Autodesk Inventor part; units mm, degrees
ref_plane "YZ Plane" through (0, 0, 0) normal (1, 0, 0) x (0, 1, 0)
ref_plane "XZ Plane" through (0, 0, 0) normal (0, 1, 0) x (-1, 0, 0)
ref_plane "XY Plane" through (0, 0, 0) normal (0, 0, 1) x (1, 0, 0)
sketch "Sketch1" plane through (0, 0, 0) normal (0, 1, 0) x (-1, 0, 0)
  line L0 (16.2, 12.4) -> (-16.2, 12.4)
  line L1 (-16.2, 12.4) -> (-16.2, -12.4)
  line L2 (-16.2, -12.4) -> (16.2, -12.4)
  line L3 (16.2, -12.4) -> (16.2, 12.4)
  line L4 (16.2, 12.4) -> (-16.2, -12.4) construction
  line L5 (-16.2, 12.4) -> (16.2, -12.4) construction
  point P0 (0, 0)
  dimension "d0" = 32.4
  dimension "d1" = 24.8
extrude "Extrusion1" add sketch "Sketch1" against normal blind 1.4
sketch "Sketch2" plane through (0, 0, 0) normal (0, 1, 0) x (1, 0, 0)
  line L0 (-18, -14) -> (18, -14)
  line L1 (18, -14) -> (18, 14)
  line L2 (18, 14) -> (-18, 14)
  line L3 (-18, 14) -> (-18, -14)
  line L4 (-18, -14) -> (18, 14) construction
  line L5 (18, -14) -> (-18, 14) construction
  point P0 (0, 0)
  dimension "d4" = 36
  dimension "d5" = 28
extrude "Extrusion2" add sketch "Sketch2" along normal blind 2
sketch "Sketch3" plane through (0, 2, 0) normal (0, 1, 0) x (1, 0, 0)
  line L0 (-8.5, -9) -> (8.5, -9)
  line L1 (8.5, -9) -> (8.5, 9)
  line L2 (8.5, 9) -> (-8.5, 9)
  line L3 (-8.5, 9) -> (-8.5, -9)
  line L4 (-8.5, -9) -> (8.5, 9) construction
  line L5 (8.5, -9) -> (-8.5, 9) construction
  circle A0 centre (-13.5, 0) radius 1.75
  circle A1 centre (13.5, 0) radius 1.75
  point P0 (0, 0)
  dimension "d8" = 17
  dimension "d9" = 18
  dimension "d10" = 13.5
  dimension "d11" = 13.5
  dimension "d12" = 3.5
  dimension "d13" = 3.5
extrude "Extrusion3" cut sketch "Sketch3" against normal up to surface (3.4 mm away)
properties part number "network panel_3DPrint"
The listing builds one solid part. Answer for the finished solid, in the listing's coordinates (mm). A direction names the side the tool comes from. Round coordinates to 2 decimals unless told otherwise and drop trailing zeros. Write each loop counter-clockwise with the first axis right and the second up, starting at its lowest first coordinate (ties: lowest second). Pieces come first, ordered by that corner, then holes. Notation, with made-up numbers: (-20.5, 68) -> (4.5, 68) arc R10 ccw to (4.5, 79) -> close; hole circle Ø1 at (60, -38.5). An arc over 180 degrees is marked (long way). Answer as a JSON object with one key per item and string values. Group by question number.
Q1. Section C-C (z = -5.5) is taken. Write down the section's boundary in (x, y).
Q2. Determine the mould class of faces 6 (the face through (8.5, 0, 0)), 7 (the face through (18, 1, 0)), 8 (the face through (0, 0, -13)) for opening direction X: pulls with the +X half, pulls with the -X half, needs draft (parallel to the pull), parting line crosses it, or undercut.
Q3. Section B-B (x = 13.5) is taken. Write down the section's boundary in (y, z).
Q4. Each of these flat-tipped pins is pushed along its axis until it touches: pin 1 Ø0.7 at (y, z) = (-0.5, 2.5) entering from -X; pin 2 Ø1.1 at (x, y) = (-2.5, -1) entering from +Z. Where does it stop, or does it pass through?
Q5. Section A-A (z = 0) is taken. Write down the section's boundary in (x, y), plus the area to 3 significant figures.
Q6. Straight lines are drawn through the part: line 1 along X through (y, z) = (-0.4, 0); line 2 along X through (y, z) = (1.3, 0); line 3 along Z through (x, y) = (0.5, -0.2). For each, find the intervals that lie inside material, in ascending order.
Q7. Which of the six approach directions +Z, -Z, +X, -X, +Y, -Y give full straight-line access (tool end or side, diameter ignored) to faces 1 (the face through (16.2, -1, 0)), 2 (the face through (0, 0, 9)), 3 (the face through (0, -1, 12.4)), 4 (the face through (0, -1, -12.4)), 5 (the face through (-16.2, -1, 0))?
Q8. Section D-D (z = -9.5) is taken. Write down the section's boundary in (x, y).
Check values:
{
 "1": {"outline": "(-18, 0) -> (-16.2, 0) -> (-16.2, -1.4) -> (-8.5, -1.4) -> (-8.5, 2) -> (-18, 2) -> close; (8.5, -1.4) -> (16.2, -1.4) -> (16.2, 0) -> (18, 0) -> (18, 2) -> (8.5, 2) -> close"},
 "2": {"face 6": "undercut", "face 7": "pulls with the +X half", "face 8": "needs draft"},
 "3": {"outline": "(-1.4, -12.4) -> (0, -12.4) -> (0, -14) -> (2, -14) -> (2, -1.75) -> (-1.4, -1.75) -> close; (-1.4, 1.75) -> (2, 1.75) -> (2, 14) -> (0, 14) -> (0, 12.4) -> (-1.4, 12.4) -> close"},
 "4": {"pin 1": "x = -16.2", "pin 2": "z = 12.4"},
 "5": {"outline": "(-18, 0) -> (-16.2, 0) -> (-16.2, -1.4) -> (-15.25, -1.4) -> (-15.25, 2) -> (-18, 2) -> close; (-11.75, -1.4) -> (-8.5, -1.4) -> (-8.5, 2) -> (-11.75, 2) -> close; (8.5, -1.4) -> (11.75, -1.4) -> (11.75, 2) -> (8.5, 2) -> close; (15.25, -1.4) -> (16.2, -1.4) -> (16.2, 0) -> (18, 0) -> (18, 2) -> (15.25, 2) -> close", "area": "35.8 mm^2"},
 "6": {"line 1": "-16.2 to -15.25, -11.75 to -8.5, 8.5 to 11.75, 15.25 to 16.2", "line 2": "-18 to -15.25, -11.75 to -8.5, 8.5 to 11.75, 15.25 to 18", "line 3": "-12.4 to -9, 9 to 12.4"},
 "7": {"face 1": "+Z, -Z, +X, -Y", "face 2": "+Y, -Y", "face 3": "+Z, +X, -X, -Y", "face 4": "-Z, +X, -X, -Y", "face 5": "+Z, -Z, -X, -Y"},
 "8": {"outline": "(-18, 0) -> (-16.2, 0) -> (-16.2, -1.4) -> (16.2, -1.4) -> (16.2, 0) -> (18, 0) -> (18, 2) -> (-18, 2) -> close"}
}
